Autodesk Inventor part; units mm, degrees
ref_plane "YZ Plane" through (0, 0, 0) normal (1, 0, 0) x (0, 1, 0)
ref_plane "XZ Plane" through (0, 0, 0) normal (0, 1, 0) x (-1, 0, 0)
ref_plane "XY Plane" through (0, 0, 0) normal (0, 0, 1) x (1, 0, 0)
sketch "Sketch1" plane through (0, 0, 0) normal (0, 0, 1) x (1, 0, 0)
  line L0 (0, 0) -> (80, 0)
  line L1 (80, 0) -> (80, 80)
  line L2 (80, 80) -> (0, 80)
  line L3 (0, 80) -> (0, 0)
  dimension "d0" = 80
  dimension "d1" = 80
extrude "Extrusion1" add sketch "Sketch1" along normal blind 60
sketch "Sketch2" plane through (0, 0, 60) normal (0, 0, 1) x (1, 0, 0)
  circle A0 centre (40, 40) radius 30
  line L0 (0, 80) -> (0, 0)
  line L1 (80, 80) -> (0, 80)
  dimension "d4" = 40
  dimension "d5" = 40
  dimension "d6" = 60
extrude "Extrusion2" add sketch "Sketch2" along normal blind 1
sketch "Sketch3" plane through (40, 40, 61) normal (0, 0, 1) x (1, 0, 0)
  circle A0 centre (0, 0) radius 12.5
  point P0 (-40, -40)
  dimension "d9" = 25
extrude "Extrusion3" add sketch "Sketch3" along normal blind 20
sketch "Sketch4" plane through (40, 40, 81) normal (0, 0, 1) x (1, 0, 0)
  circle A0 centre (0, 0) radius 22.5
  point P0 (-40, -40)
  dimension "d12" = 45
extrude "Extrusion4" add sketch "Sketch4" along normal blind 10
fillet "Fillet1" radius 20 1 edges at (17.5, 40, 91)
properties part number "emergencyStop"
Source: CAD feature listing. Evaluate the final solid. Frame: model axes, mm. A direction names the side the tool comes from. Give positions to 0.01 mm unless a question says otherwise; leave off trailing zeros. Order: outer loops, then holes, each group sorted by start corner. A loop starts at its lowest first (then second) coordinate and runs counter-clockwise, first axis right, second up. Notation, with made-up numbers: (-1.75, -7) -> (22.25, -7) arc R16 cw to (22.25, 24) -> close; hole circle Ø3 at (78.5, 83.5). An arc over 180 degrees is marked (long way). Write item = value, one per line.
Q1. Material intervals for line 1 (Z direction, x = 66, y = 64); line 2 (Z direction, x = 32, y = 25.5); line 3 (Z direction, x = 17, y = 59), sorted ascending. Write a range as from..to.
Data:
line_1 = 0..60
line_2 = 0..61, 81..87.45
line_3 = 0..61
Q2. Cut plane A-A, the plane x = 66.5. Output: boundary loops of the cut face in (y, z), and give its area (3 significant figures).
Data:
outline = (0, 0) -> (80, 0) -> (80, 60) -> (54.06, 60) -> (54.06, 61) -> (25.94, 61) -> (25.94, 60) -> (0, 60) -> close
area = 4,830 mm^2
Q3. Pin query (flat end, axial travel): pin 1 (2 mm diameter, centred on x = 38, z = 78.5, fed in from +Y); pin 2 (10 mm diameter, centred on x = 18, z = 75, fed in from -Y); pin 3 (1 mm diameter, centred on x = 18.5, y = 66, fed in from +Z); pin 4 (10 mm diameter, centred on x = 41, y = 68, fed in from +Z). Return the tip coordinate at first contact, or that it passes through.
Data:
pin_1 = 52.46
pin_2 = through
pin_3 = 60
pin_4 = 61
Q4. Pull-direction query (Z, two-part tool) for faces 1 (the face through (30.08, 47.606, 70.86)), 2 (the face through (53, 40, 61)), 3 (the face through (22, 67, 60)), 4 (the face through (39, 41, 0)); classes: released by +Z, released by -Z, zero draft, split by the parting line, or undercut.
Data:
face_1 = undercut
face_2 = undercut
face_3 = released by +Z
face_4 = released by -Z
Q5. Set-up query: faces 5 (the face through (33.497, 69.287, 60.493)), 6 (the face through (0, 41, 30)), 7 (the face through (50, 30, 81)). Return all of +Z, -Z, +X, -X, +Y, -Y with unobstructed straight access to the full face (end or side cutting, diameter ignored); none if empty.
Data:
face_5 = +Z
face_6 = +Z, -Z, -X, +Y, -Y
face_7 = none
